Autodesk Inventor part; units mm, degrees
ref_plane "YZ Plane" through (0, 0, 0) normal (1, 0, 0) x (0, 1, 0)
ref_plane "XZ Plane" through (0, 0, 0) normal (0, 1, 0) x (-1, 0, 0)
ref_plane "XY Plane" through (0, 0, 0) normal (0, 0, 1) x (1, 0, 0)
sketch "Sketch1" plane through (0, 0, 0) normal (0, 1, 0) x (-1, 0, 0)
  line L0 (-7.5, 0) -> (7.5, 0)
  line L1 (7.5, 0) -> (7.5, -30)
  line L2 (7.5, -30) -> (13, -30)
  line L3 (13, -30) -> (13, 40)
  line L4 (13, 40) -> (-13, 40)
  line L5 (-13, 40) -> (-13, -30)
  line L6 (-13, -30) -> (-7.5, -30)
  line L7 (-7.5, -30) -> (-7.5, 0)
  line L8 (0, 0) -> (0, 40) construction
  line L9 (-11, 8) -> (11, 8) construction
  point P0 (0, 8)
  dimension "d0" = 22
  dimension "d1" = 30
  dimension "d2" = 15
  dimension "d3" = 8
  dimension "d8" = 26
  dimension "d9" = 40
extrude "Extrusion1" add sketch "Sketch1" along normal blind 26
sketch "Sketch2" plane through (13, 0, 40) normal (1, 0, 0) x (0, 0, -1)
  line L0 (70, 0) -> (70, 26)
  circle A0 centre (57, 13) radius 4
  point P0 (40, 0)
  point P1 (70, 13)
  dimension "d10" = 8
  dimension "d11" = 13
extrude "Extrusion2" cut sketch "Sketch2" against normal up to surface (26 mm away)
fillet "Fillet1" radius 13 4 edges at (-10.25, 26, -30) (10.25, 26, -30) (-10.25, 0, -30) (10.25, 0, -30)
sketch "Sketch3" plane through (-13, 0, 40) normal (0, 0, 1) x (1, 0, 0)
  line L0 (0, 0) -> (26, 0)
  line L1 (26, 0) -> (26, 26)
  circle A0 centre (13, 13) radius 11
  point P0 (13, 0)
  point P1 (26, 13)
  point P2 (13, 0)
  dimension "d15" = 22
extrude "Extrusion3" cut sketch "Sketch3" against normal blind 35
sketch "Sketch4" plane through (7.5, 0, 0) normal (-1, 0, 0) x (0, 0, 1)
  arc A0 (-17, 26) -> (-17, 0) centre (-17, 13) ccw
  line L0 (-17, 0) -> (0, 0)
  line L1 (0, 0) -> (0, 26)
  line L2 (-17, 26) -> (0, 26)
  arc A1 (0, 13) -> (-6.0455, 26) centre (-17, 13) ccw
  arc A2 (-6.1134, -0.0569) -> (0, 13) centre (-17, 13) ccw
  line L3 (-6.0455, 0) -> (0, 0)
  line L4 (0, 26) -> (-6.0455, 26)
  circle A3 centre (-17, 13) radius 4
  circle A4 centre (-17, 13) radius 13 construction
  line L5 (-4, 23.9545) -> (-4, 2.0455) construction
  line L6 (-4, 23.9545) -> (-4, 26)
  line L7 (-4, 2.0455) -> (-4, 0)
extrude "Extrusion5" add sketch "Sketch4" along normal up to next contours L2 L1 A1 L6 | L7 A2 L1 L0
properties part number "spoke"
Geometry check sheet. Reference: the model listing, model coordinates, mm. A direction names the side the tool comes from. Coordinates: 2 decimals unless noted, no trailing zeros. Loops run counter-clockwise (first coordinate to the right, second up) from the corner with the lowest first, then second, coordinate; pieces in that order, holes last. Notation, with made-up numbers: (-6, 62) -> (28, 62) arc R17 cw to (28, 66) -> close; hole circle Ø4 at (57.25, 45.5). An arc over 180 degrees is marked (long way). Put each result on its own line as item: value.
1) Cross-section at D-D on z = 13. Record the boundary of the cut face in (x, y).
Result set:
outline: (-13, 0) -> (13, 0) -> (13, 26) -> (-13, 26) -> close; hole circle Ø22 at (0, 13)
2) Thickness scan on line 1 (X direction, y = 18, z = -12.5); line 2 (Y direction, x = -10.95, z = -17); line 3 (Y direction, x = 0, z = 18). Record the ranges inside material, lowest first.
Result set:
line 1: x = -13 to -7.5, 7.5 to 13
line 2: y = 0 to 9, 17 to 26
line 3: y = 0 to 2, 24 to 26
3) Cross-section at A-A on z = -8.5. Record the boundary of the cut face in (x, y), plus the area to 3 significant figures.
Result set:
outline: (-13, 0) -> (-7.5, 0) -> (-7.5, 26) -> (-13, 26) -> close; (7.5, 0) -> (13, 0) -> (13, 26) -> (7.5, 26) -> close
area: 286 mm^2
4) Cross-section at C-C on x = 0. Record the boundary of the cut face in (y, z).
Result set:
outline: (0, -4) -> (2.05, -4) arc R17 cw to (13, 0) arc R17 cw to (23.95, -4) -> (26, -4) -> (26, 40) -> (24, 40) -> (24, 5) -> (2, 5) -> (2, 40) -> (0, 40) -> close
5) Tool access check on faces 4 (the flat face through (0, 25, -4)), 5 (the cylindrical face through (-2.38, 2.26, 22.74)), 6 (the cylindrical face through (0.11, 18.91, -1.06)), 7 (the flat face through (-13, 13, 5)). Record the directions out of +Z, -Z, +X, -X, +Y, -Y that give a thin tool (end or side, any length) a straight path to the whole face; none if there is none.
Result set:
face 4: -Z, +Y, -Y
face 5: +Z
face 6: -Z
face 7: +Z, -Z, -X, +Y, -Y
6) Cross-section at B-B on y = 14. Record the boundary of the cut face in (x, z), plus the area to 3 significant figures.
Result set:
outline: (-13, -29.96) -> (-7.5, -29.96) -> (-7.5, -20.87) -> (-13, -20.87) -> close; (-13, -13.13) -> (-7.5, -13.13) -> (-7.5, -0.03) -> (7.5, -0.03) -> (7.5, -13.13) -> (13, -13.13) -> (13, 40) -> (10.95, 40) -> (10.95, 5) -> (-10.95, 5) -> (-10.95, 40) -> (-13, 40) -> close; (7.5, -29.96) -> (13, -29.96) -> (13, -20.87) -> (7.5, -20.87) -> close
area: 518 mm^2
7) Gauge pin test, flat ends, axial feed: pin 1 Ø3 at (x, y) = (-5, 9.5) entering from +Z; pin 2 Ø2 at (x, y) = (-1.5, 9) entering from -Z; pin 3 Ø1 at (x, y) = (-0.5, 0.5) entering from -Z. Record the tip position at first contact, or that the pin passes through.
Result set:
pin 1: stops at z = 5
pin 2: stops at z = -0.75
pin 3: stops at z = -4
8) Release check for a two-part mould opening along Z. For faces 1 (the cylindrical face through (-10.21, 15.7, -14.05)), 2 (the flat face through (7.5, 13, -12)), 3 (the cylindrical face through (-10.288, 22.293, -26.091)) record: released by +Z, released by -Z, zero draft, split by the parting line, or undercut.
Result set:
face 1: undercut
face 2: zero draft
face 3: released by -Z
